Part model, mm, in its own coordinate system. A direction names the side the tool comes from. Give positions to 0.01 mm unless a question says otherwise; leave off trailing zeros. Loops run counter-clockwise (first coordinate to the right, second up) from the corner with the lowest first, then second, coordinate; pieces in that order, holes last. Notation, with made-up numbers: M -8.75,10 L 42.25,10 A27 cw 42.25,35 Z; hole C -10.5,-36 d3. An arc over 180 degrees is marked long. Put each result on its own line as item: value. Start each with the question number.
```python
from build123d import *

# Parameters (mm, degrees)
F0_W          = 79.5706696808
F0_H          = 54.8370443285
F1_DEPTH      = 25.4
F2_R          = 10.632312462
F3_DEPTH      = 25.4
F5_DEPTH      = 27.178
F5_DEPTH_BACK = 32.766


with BuildPart() as f1:
    # F0 (on Top) → F1 (new body)
    with BuildSketch(Plane.XY):
        with Locations((-11.0720153898, 5.5851843208)):
            Rectangle(F0_W, F0_H)
    extrude(amount=F1_DEPTH)

    # F2 (on face) → F3 (join)
    with BuildSketch(Plane.XY.offset(25.4)):
        with Locations((-12.4944150448, 8.600234054)):
            Circle(F2_R)
    extrude(amount=F3_DEPTH)

    # F4 (on Front) → F5 (cut, two sides)
    with BuildSketch(Plane.XZ) as f5_sk:
        Polygon((-1.411169651, 50.8574359119), (-23.2553649694, 50.8574359119), (-1.411169651, 40.8576503396), align=None)
    extrude(amount=-F5_DEPTH, mode=Mode.SUBTRACT)
    extrude(f5_sk.sketch, amount=F5_DEPTH_BACK, mode=Mode.SUBTRACT)


solid = f1.part
```
1) Pin check, flat tips, straight feed: pin 1 Ø6 at (x, y) = (-29, 20) entering from +Z; pin 2 Ø8 at (x, y) = (0, 8) entering from -Z. Stop position of each tip, or through.
2) Band-saw the part on B-B on y = -8. Give the cut face in (x, z).
3) Band-saw the part on A-A on x = -39. Give the cut face in (y, z).
4) Band-saw the part on D-D on x = -13. Give the cut face in (y, z).
5) Which spindle directions (+Z, -Z, +X, -X, +Y, -Y) get a long thin tool onto all of the face, cutting with end or side? Do faces 1 (the cylindrical face through (-23.116, 9.068, 35.176)), 2 (the flat face through (-12, 33.004, 13)). Say none if no direction does.
6) Wall check: L1, parallel to Z at x = -15, y = 25; L2, parallel to X at y = 8.5, z = 35.5; L3, parallel to Y at x = -7, z = 28.5. Give the ranges that are in metal, low to high.
7) Band-saw the part on C-C on z = 39.5. Give the cut face in (x, y), then the cut area to 3 significant figures.
Evaluation:
1. pin 1: z = 25.4
1. pin 2: z = 0
2. outline: M -50.86,0 L 28.71,0 L 28.71,25.4 L -50.86,25.4 Z
3. outline: M -21.83,0 L 33,0 L 33,25.4 L -21.83,25.4 Z
4. outline: M -21.83,0 L 33,0 L 33,25.4 L 19.22,25.4 L 19.22,46.16 L -2.02,46.16 L -2.02,25.4 L -21.83,25.4 Z
5. face 1: +Z
5. face 2: +Z, -Z, +X, -X, +Y
6. L1: 0 to 25.4
6. L2: -23.13 to -1.86
6. L3: -0.5 to 17.7
7. outline: C -12.49,8.6 d21.26
7. area: 355 mm2
